```python
from build123d import *

# Parameters (mm, degrees)
SKETCH1_R           = 7.5
SKETCH1_R_2         = 12.5
SKETCH1_R_3         = 3
BOSS_EXTRUDE1_DEPTH = 7


with BuildPart() as part:
    # Sketch1 → Boss-Extrude1 (new body)
    with BuildSketch(Plane.XY):
        with BuildLine():
            Line((-54.759819531, 6.565702497), (-16.759819531, 103.565702497))
            ThreePointArc((-16.759819531, 103.565702497), (0, 115), (16.759819531, 103.565702497))
            Line((16.759819531, 103.565702497), (54.759819531, 6.565702497))
            ThreePointArc((54.759819531, 6.565702497), (52.869139937, -10.144391432), (38, -18))
            Line((38, -18), (-38, -18))
            ThreePointArc((-38, -18), (-52.869139937, -10.144391432), (-54.759819531, 6.565702497))
        make_face()
        with Locations((0, 97)):
            Circle(SKETCH1_R, mode=Mode.SUBTRACT)
        with Locations((-38, 0)):
            Circle(SKETCH1_R, mode=Mode.SUBTRACT)
        with Locations((38, 0)):
            Circle(SKETCH1_R, mode=Mode.SUBTRACT)
        with Locations((0, 14)):
            Circle(SKETCH1_R_2, mode=Mode.SUBTRACT)
        with Locations((0, -3.5)):
            Circle(SKETCH1_R_3, mode=Mode.SUBTRACT)
        with Locations((-15.155444566, 22.75)):
            Circle(SKETCH1_R_3, mode=Mode.SUBTRACT)
        with Locations((15.155444566, 22.75)):
            Circle(SKETCH1_R_3, mode=Mode.SUBTRACT)
    extrude(amount=BOSS_EXTRUDE1_DEPTH)


solid = part.part
```
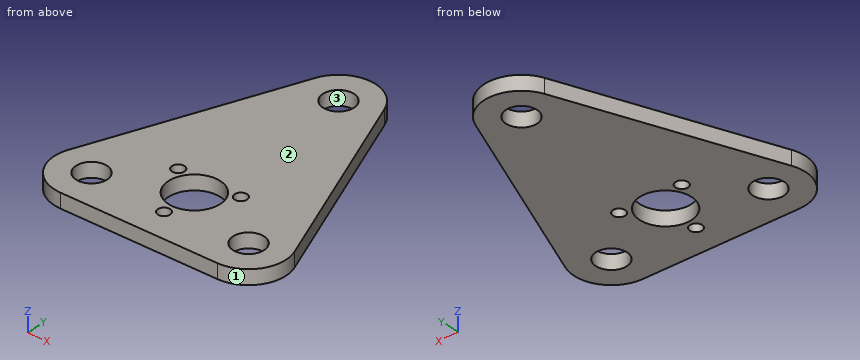
Design review of the part built by this model. Coordinates are the model's own, in mm. Face numbers are marked on the shaded views. Give positions to 0.01 mm unless a question says otherwise; leave off trailing zeros. Order: outer loops, then holes, each group sorted by start corner. A loop starts at its lowest first (then second) coordinate and runs counter-clockwise, first axis right, second up. Notation, with made-up numbers: (73.25, 86.25) -> (77.25, 86.25) arc R31 cw to (77.25, 125.25) -> close; hole circle Ø10 at (77, 89). An arc over 180 degrees is marked (long way). Write item = value, one per line. Start each with the question number.
(1) We need section A-A on x = 0. Write out the cut boundary in (y, z), plus the area to 3 significant figures.
(2) For pin 1 (6 mm diameter, centred on x = -38.5, y = 61, fed in from +Z); pin 2 (3 mm diameter, centred on y = -4, z = 2.5, fed in from +X); pin 3 (1.5 mm diameter, centred on y = 74, z = 2.5, fed in from +X), all flat-tipped, find the tip position at first contact; note any pin that passes through.
(3) To check wall thickness, follow line 1 along X through (y, z) = (102.5, 2.25); line 2 along X through (y, z) = (11.5, 3.75); line 3 along X through (y, z) = (-9.5, 3.5). State the ranges of each line that lie inside material, in increasing order.
(4) We need section B-B on z = 3.75. Write out the cut boundary in (x, y).
(5) We need section D-D on y = -3.5. Write out the cut boundary in (x, z).
(6) Mouldability with a two-part tool opening along Y and no side actions: class the marked faces 1, 2 and 3 as +Y half, -Y half, draft (parallel to the pull), parting line (faces both ways), or undercut.
(7) We need section C-C on y = 14. Write out the cut boundary in (x, z).
Numbers:
q1.outline = (-18, 0) -> (-6.5, 0) -> (-6.5, 7) -> (-18, 7) -> close; (-0.5, 0) -> (1.5, 0) -> (1.5, 7) -> (-0.5, 7) -> close; (26.5, 0) -> (89.5, 0) -> (89.5, 7) -> (26.5, 7) -> close; (104.5, 0) -> (115, 0) -> (115, 7) -> (104.5, 7) -> close
q1.area = 609 mm^2
q2.pin_1 = through
q2.pin_2 = 55.83
q2.pin_3 = 28.64
q3.line_1 = -17.18 to -5.1, 5.1 to 17.18
q3.line_2 = -52.83 to -12.25, 12.25 to 52.83
q3.line_3 = -53.29 to 53.29
q4.outline = (-54.76, 6.57) arc R18 ccw to (-38, -18) -> (38, -18) arc R18 ccw to (54.76, 6.57) -> (16.76, 103.57) arc R18 ccw to (-16.76, 103.57) -> close; hole circle Ø15 at (-38, 0); hole circle Ø6 at (-15.16, 22.75); hole circle Ø25 at (0, 14); hole circle Ø15 at (0, 97); hole circle Ø6 at (0, -3.5); hole circle Ø6 at (15.16, 22.75); hole circle Ø15 at (38, 0)
q5.outline = (-55.66, 0) -> (-44.63, 0) -> (-44.63, 7) -> (-55.66, 7) -> close; (-31.37, 0) -> (-3, 0) -> (-3, 7) -> (-31.37, 7) -> close; (3, 0) -> (31.37, 0) -> (31.37, 7) -> (3, 7) -> close; (44.63, 0) -> (55.66, 0) -> (55.66, 7) -> (44.63, 7) -> close
q6.face_1 = parting line
q6.face_2 = draft
q6.face_3 = undercut
q7.outline = (-51.85, 0) -> (-12.5, 0) -> (-12.5, 7) -> (-51.85, 7) -> close; (12.5, 0) -> (51.85, 0) -> (51.85, 7) -> (12.5, 7) -> close
